Autodesk Inventor part; units mm, degrees
ref_plane "Work Plane1" through (0, 0, 91.44) normal (0, 0, 1) x (1, 0, 0)
ref_plane "YZ Plane" through (0, 0, 0) normal (1, 0, 0) x (0, 1, 0)
ref_plane "XZ Plane" through (0, 0, 0) normal (0, 1, 0) x (-1, 0, 0)
sketch "Sketch1" plane through (0, 0, 0) normal (0, 0, 1) x (1, 0, 0)
  circle A0 centre (0, 0) radius 34.925
  dimension "d0" = 69.85
extrude "Extrusion1" add sketch "Sketch1" along normal blind 63.5
sketch "Sketch2" plane through (0, 0, 63.5) normal (0, 0, 1) x (1, 0, 0)
  circle A0 centre (0, 0) radius 22.225
  dimension "d3" = 44.45
extrude "Extrusion2" add sketch "Sketch2" along normal blind 12.7
sketch "Sketch3" plane through (0, 0, 76.2) normal (0, 0, 1) x (1, 0, 0)
  circle A0 centre (0, 0) radius 9.525
  dimension "d6" = 19.05
extrude "Extrusion3" add sketch "Sketch3" along normal blind 2.54
sketch "Sketch4" plane through (0, 0, 78.74) normal (0, 0, 1) x (1, 0, 0)
  circle A0 centre (0, 0) radius 2.3729
extrude "Extrusion4" add sketch "Sketch4" along normal blind 12.7
ref_plane "Work Plane1" through (0, 0, 91.44) normal (0, 0, 1) x (1, 0, 0)
sketch "Sketch5" plane through (0, 0, 91.44) normal (0, 0, 1) x (1, 0, 0)
  circle A0 centre (0, 0) radius 3.9381
extrude "Extrusion5" add sketch "Sketch5" against normal blind 1.27
sketch "Sketch6" plane through (0, 0, 78.74) normal (0, 0, 1) x (1, 0, 0)
  line L0 (0, 0) -> (-16.51, 0)
  circle A0 centre (-16.51, 0) radius 2.54
  dimension "d14" = 16.51
  dimension "d15" = 5.08
extrude "Extrusion6" cut sketch "Sketch6" against normal blind 38.1
sketch "Sketch7" plane through (0, 0, 76.2) normal (0, 0, 1) x (1, 0, 0)
  line L0 (0, 0) -> (16.51, 0)
  circle A0 centre (16.51, 0) radius 2.54
  dimension "d18" = 16.51
  dimension "d19" = 5.08
extrude "Extrusion7" cut sketch "Sketch7" against normal blind 38.1
sketch "Sketch8" plane through (0, 0, 0) normal (0, 0, -1) x (-1, 0, 0)
  circle A0 centre (0, 0) radius 31.0151
extrude "Extrusion8" cut sketch "Sketch8" against normal blind 50.8
sketch "Sketch9" plane through (0, 0, 0) normal (0, 0, -1) x (-1, 0, 0)
  circle A0 centre (0, 0) radius 34.925
extrude "Extrusion9" add sketch "Sketch9" along normal blind 0.254
properties part number "000109"
Here's how the part is built. I have some questions about the finished solid (model axes, mm). A direction names the side the tool comes from. Round coordinates to 2 decimals unless told otherwise and drop trailing zeros. Loops run counter-clockwise (first coordinate to the right, second up) from the corner with the lowest first, then second, coordinate; pieces in that order, holes last.
1. If we section it at C-C on z = 62: Write out the boundary of the cut face in (x, y) (3 decimals).
Answer list:
outline: circle Ø69.85 at (0, 0); hole circle Ø5.08 at (-16.51, 0); hole circle Ø5.08 at (16.51, 0)
2. We'd pull the mould along X, two halves only. Please class faces 1 (the face through (0, 0, 50.8)), 2 (the face through (2, -2, 90.17)), 3 (the face through (-0.854, -3.844, 90.814)): +X half, -X half, draft (parallel to the pull), parting line (faces both ways), or undercut.
Answer list:
face 1: undercut
face 2: draft
face 3: parting line
3. For P1, Ø10, axis at y = 16.5, z = 57.5, coming from the -X side; P2, Ø21, axis at x = 14, y = 1.5, coming from the +Z side; P3, Ø5, axis at x = -10.5, z = 24, coming from the +Y side; P4, Ø1.5, axis at y = 20, z = 61.5, coming from the -X side, each with a flat end and sliding along its axis, tell me the tip position at first contact or that it passes through.
Answer list:
P1: stops at x = -32.98
P2: stops at z = 91.44
P3: stops at y = 34
P4: stops at x = -29.14
4. If I drill on line 1 along Z through (x, y) = (-19, 24); line 2 along Z through (x, y) = (-9.5, 16); line 3 along Y through (x, z) = (0, 26) (3 decimals), over which ranges is the centre line in solid material (lowest first)?
Answer list:
line 1: z = -0.25 to 0, 50.8 to 63.5
line 2: z = -0.25 to 0, 50.8 to 76.2
line 3: y = -34.925 to -31.015, 31.015 to 34.925
5. If we section it at B-B on x = 0: Write out the boundary of the cut face in (y, z) (3 decimals), plus the area to 3 significant figures.
Answer list:
outline: (-34.925, -0.254) - (34.925, -0.254) - (34.925, 63.5) - (22.225, 63.5) - (22.225, 76.2) - (9.525, 76.2) - (9.525, 78.74) - (2.373, 78.74) - (2.373, 90.17) - (3.938, 90.17) - (3.938, 91.44) - (-3.938, 91.44) - (-3.938, 90.17) - (-2.373, 90.17) - (-2.373, 78.74) - (-9.525, 78.74) - (-9.525, 76.2) - (-22.225, 76.2) - (-22.225, 63.5) - (-34.925, 63.5) - close; hole (-31.015, 0) - (31.015, 0) - (31.015, 50.8) - (-31.015, 50.8) - close
area: 1,980 mm2
6. If we section it at D-D on y = -14: Write out the boundary of the cut face in (x, z), plus the area to 3 significant figures.
Answer list:
outline: (-32, -0.25) - (32, -0.25) - (32, 63.5) - (17.26, 63.5) - (17.26, 76.2) - (-17.26, 76.2) - (-17.26, 63.5) - (-32, 63.5) - close; hole (-27.68, 0) - (27.68, 0) - (27.68, 50.8) - (-27.68, 50.8) - close
area: 1,710 mm2
7. Which directions (+Z, -Z, +X, -X, +Y, -Y) give clear straight access to the entire face, cutting with the end or side of a thin tool? Please do faces 4 (the face through (18.856, -0.973, 63.678)), 5 (the face through (24.613, -18.872, 25.044)), 6 (the face through (0, 0, -0.254)).
Answer list:
face 4: +Z
face 5: none
face 6: -Z, +X, -X, +Y, -Y
